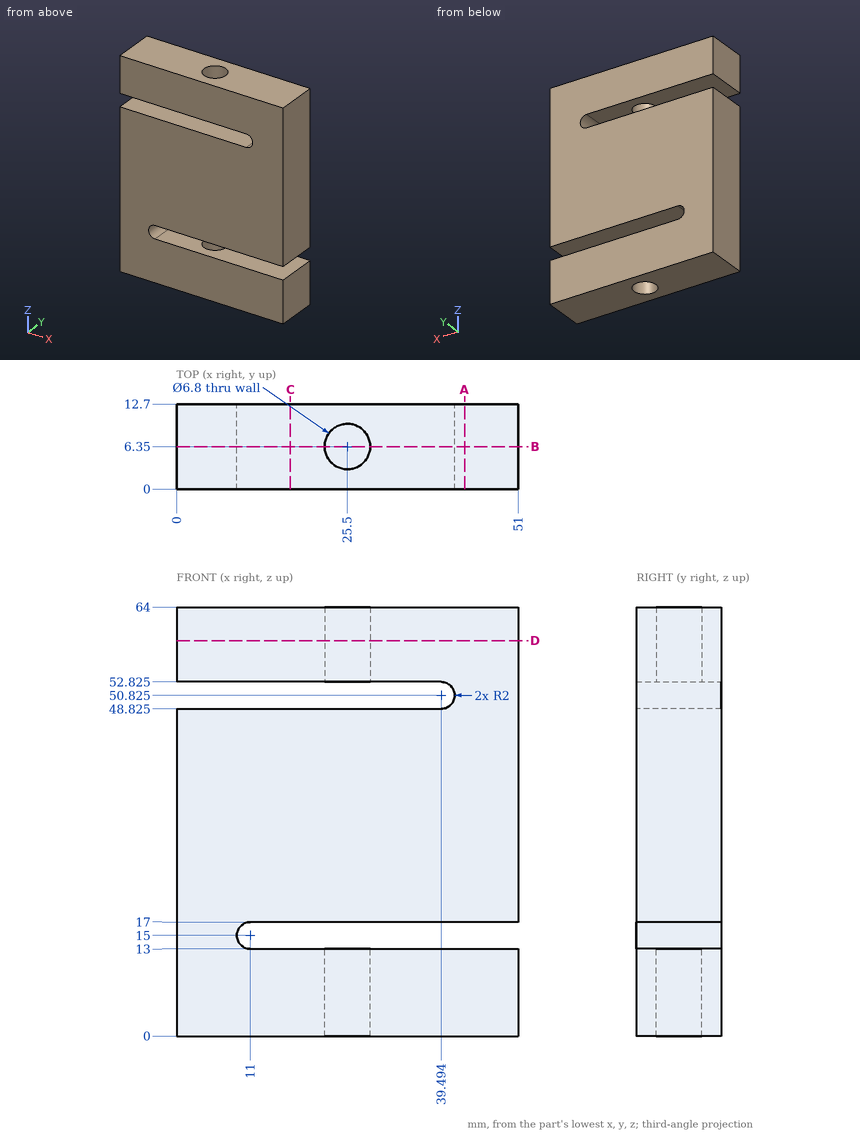
For this review, use the dimensioned drawing (mm, ordinates from the lowest corner) and the shaded views. Round coordinates to 2 decimals unless told otherwise and drop trailing zeros. Write each loop counter-clockwise with the first axis right and the second up, starting at its lowest first coordinate (ties: lowest second). Pieces come first, ordered by that corner, then holes. Notation, with made-up numbers: (26, 3.5) -> (65, 3.5) arc R36 cw to (65, 42.5) -> close; hole circle Ø3 at (63.25, -9.75). An arc over 180 degrees is marked (long way). One line per item, written item: value. Start each with the question number.
Q1. Add section B-B (y = 6.35). Give the boundary of the cut face in (x, z) (3 decimals).
Q2. Insertion check: P1, Ø6.5, axis at x = 22.5, y = 7, coming from the -Z side. The pin has a flat end and moves straight along its axis. Give the tip position at first contact, or say it passes through.
Q3. Add section A-A (x = 43). Give the boundary of the cut face in (y, z).
Q4. Add section D-D (z = 59). Give the boundary of the cut face in (x, y), then the cut area to 3 significant figures.
Q5. To check wall thickness, follow probe 1 along Z at (x, y) = (36.5, 3) (3 decimals); probe 2 along Z at (x, y) = (5.5, 8.25) (3 decimals); probe 3 along Z at (x, y) = (47.5, 9). State the ranges of each line that lie inside material, in increasing order.
Q6. Add section C-C (x = 17). Give the boundary of the cut face in (y, z) (3 decimals).
Response:
1. outline: (0, 0) -> (22.1, 0) -> (22.1, 13) -> (11, 13) arc R2 cw to (11, 17) -> (51, 17) -> (51, 64) -> (28.9, 64) -> (28.9, 52.825) -> (39.494, 52.825) arc R2 cw to (39.494, 48.825) -> (0, 48.825) -> close; (0, 52.825) -> (22.1, 52.825) -> (22.1, 64) -> (0, 64) -> close; (28.9, 0) -> (51, 0) -> (51, 13) -> (28.9, 13) -> close
2. P1: stops at z = 0
3. outline: (0, 0) -> (12.7, 0) -> (12.7, 13) -> (0, 13) -> close; (0, 17) -> (12.7, 17) -> (12.7, 64) -> (0, 64) -> close
4. outline: (0, 0) -> (51, 0) -> (51, 12.7) -> (0, 12.7) -> close; hole circle Ø6.8 at (25.5, 6.35)
4. area: 611 mm^2
5. probe 1: z = 0 to 13, 17 to 48.825, 52.825 to 64
5. probe 2: z = 0 to 48.825, 52.825 to 64
5. probe 3: z = 0 to 13, 17 to 64
6. outline: (0, 0) -> (12.7, 0) -> (12.7, 13) -> (0, 13) -> close; (0, 17) -> (12.7, 17) -> (12.7, 48.825) -> (0, 48.825) -> close; (0, 52.825) -> (12.7, 52.825) -> (12.7, 64) -> (0, 64) -> close
